For this review, take the finished solid that the model builds, in its own axes (mm). A direction names the side the tool comes from. Round coordinates to 2 decimals unless told otherwise and drop trailing zeros. Write each loop counter-clockwise with the first axis right and the second up, starting at its lowest first coordinate (ties: lowest second). Pieces come first, ordered by that corner, then holes. Notation, with made-up numbers: (32, 14.25) -> (73, 14.25) arc R13 ccw to (73, 34.25) -> close; hole circle Ø4 at (-29.5, 17.25). An arc over 180 degrees is marked (long way). Answer in a Markdown table with one row per item. Add a question column.
```python
from build123d import *

# Parameters (mm, degrees)
SKETCH1_R           = 5
BOSS_EXTRUDE1_DEPTH = 150
SKETCH2_W           = 50
SKETCH2_H           = 20
BOSS_EXTRUDE2_DEPTH = 10
SKETCH3_R           = 5
BOSS_EXTRUDE3_DEPTH = 30
BOSS_EXTRUDE4_DEPTH = 10
SKETCH5_R           = 2.5
BOSS_EXTRUDE5_DEPTH = 250


with BuildPart() as part:
    # Sketch1 → Boss-Extrude1 (new body)
    with BuildSketch(Plane(origin=(0, 0, 0), x_dir=(1, 0, 0), z_dir=(0, 1, 0))):
        with Locations(Location((0, 0, 0), (0, 0, 270))):
            Circle(SKETCH1_R)
    extrude(amount=BOSS_EXTRUDE1_DEPTH)

    # Sketch2 → Boss-Extrude2 (add)
    with BuildSketch(Plane(origin=(0, 150, 0), x_dir=(1, 0, 0), z_dir=(0, 1, 0))):
        Rectangle(SKETCH2_W, SKETCH2_H)
    extrude(amount=BOSS_EXTRUDE2_DEPTH)

    # Sketch3 → Boss-Extrude3 (add)
    with BuildSketch(Plane(origin=(0, 160, 0), x_dir=(1, 0, 0), z_dir=(0, 1, 0))):
        with Locations(Location((-19, 0, 0), (0, 0, 270))):
            Circle(SKETCH3_R)
        with Locations(Location((19, 0, 0), (0, 0, 270))):
            Circle(SKETCH3_R)
    extrude(amount=BOSS_EXTRUDE3_DEPTH)

    # Sketch4 → Boss-Extrude4 (add)
    with BuildSketch(Plane(origin=(0, 160, 0), x_dir=(1, 0, 0), z_dir=(0, 1, 0))):
        with BuildLine():
            Line((-15, 10), (15, 10))
            ThreePointArc((15, 10), (0, 25), (-15, 10))
        make_face()
    extrude(amount=-BOSS_EXTRUDE4_DEPTH)

    # Sketch5 → Boss-Extrude5 (add)
    with BuildSketch(Plane(origin=(0, 160, 0), x_dir=(1, 0, 0), z_dir=(0, 1, 0))):
        with Locations(Location((0, 18, 0), (0, 0, 270))):
            Circle(SKETCH5_R)
    extrude(amount=-BOSS_EXTRUDE5_DEPTH)


solid = part.part
```
1. Tool access review of faces 1 (the flat face through (-20, 155, -10)), 2 (the flat face through (0, 0, 0)), 3 (the cylindrical face through (-23.88, 174.79, -1.08)), 4 (the flat face through (0, 155, 10)), 5 (the cylindrical face through (-4.88, 73.95, -1.08)): name each direction out of +Z, -Z, +X, -X, +Y, -Y from which nothing blocks a thin tool from reaching the whole face with its end or side.
2. The part is to be moulded in two halves that separate along Z. For faces 6 (the flat face through (20, 155, -10)), 7 (the cylindrical face through (0.1, 31.7, -20.5)), 8 (the flat face through (-25, 155, 0)), say which applies: pulls with the +Z half, pulls with the -Z half, needs draft (parallel to the pull), parting line crosses it, or undercut.
3. We need section A-A (x = -19). Write out the cut boundary in (y, z).
4. For L1, parallel to Y at x = 1, z = -6; L2, parallel to Y at x = 16, z = -2.5; L3, parallel to Z at x = 16, y = 161, list the stretches that pass through material, from the lowest coordinate up. Write a range as [from, to].
5. We need section B-B (y = 153). Write out the cut boundary in (x, z).
6. Clearance check with flat-ended pins moving along their axes: pin 1 Ø2 at (x, z) = (-8.5, -7) entering from -Y; pin 2 Ø12 at (x, z) = (3, -20) entering from +Y; pin 3 Ø11 at (x, z) = (2.5, -1) entering from -Y. State where each tip first meets the part, or that it passes through.
7. We need section C-C (z = 0). Write out the cut boundary in (x, y), plus the area to 3 significant figures.
8. We need section D-D (y = 95). Write out the cut boundary in (x, z).
Response:
| question | item | result |
|---|---|---|
| 1 | face 1 | -Z, -X, +Y, -Y |
| 1 | face 2 | +Z, +X, -X, -Y |
| 1 | face 3 | +Y |
| 1 | face 4 | +Z, +X, -X, +Y, -Y |
| 1 | face 5 | -Y |
| 2 | face 6 | pulls with the -Z half |
| 2 | face 7 | undercut |
| 2 | face 8 | needs draft |
| 3 | outline | (150, -10) -> (160, -10) -> (160, -5) -> (190, -5) -> (190, 5) -> (160, 5) -> (160, 10) -> (150, 10) -> close |
| 4 | L1 | [150, 160] |
| 4 | L2 | [150, 190] |
| 4 | L3 | [-4, 4] |
| 5 | outline | (-25, -10) -> (-15, -10) arc R15 ccw to (15, -10) -> (25, -10) -> (25, 10) -> (-25, 10) -> close |
| 6 | pin 1 | y = 150 |
| 6 | pin 2 | y = 160 |
| 6 | pin 3 | y = 0 |
| 7 | outline | (-25, 150) -> (-5, 150) -> (-5, 0) -> (5, 0) -> (5, 150) -> (25, 150) -> (25, 160) -> (24, 160) -> (24, 190) -> (14, 190) -> (14, 160) -> (-14, 160) -> (-14, 190) -> (-24, 190) -> (-24, 160) -> (-25, 160) -> close |
| 7 | area | 2,600 mm2 |
| 8 | outline | circle Ø10 at (0, 0); circle Ø5 at (0, -18) |
